Here's how the part is built. I have some questions about the finished solid (model axes, mm). A direction names the side the tool comes from. Round coordinates to 2 decimals unless told otherwise and drop trailing zeros. Write each loop counter-clockwise with the first axis right and the second up, starting at its lowest first coordinate (ties: lowest second). Pieces come first, ordered by that corner, then holes. Notation, with made-up numbers: (2, 35.5) - (29, 35.5) arc R27 cw to (29, 62.5) - close; hole circle Ø5 at (-18, -12). An arc over 180 degrees is marked (long way). One line per item, written item: value. Start each with the question number.
Item 1: For P1, Ø4.5, axis at x = -12.55, y = 36.5, coming from the +Z side; P2, Ø4, axis at x = 18.95, z = 389.69, coming from the +Y side; P3, Ø2.5, axis at y = 75, z = 389.69, coming from the +X side; P4, Ø1, axis at y = 26, z = 388.5, coming from the +X side, each with a flat end and sliding along its axis, tell me the tip position at first contact or that it passes through.
Item 2: Thinking about a two-plate mould opening in Z: for faces 1 (the face through (-1, 49, 384.692)), 2 (the face through (-15.48, 72.6, 389.62)), 3 (the face through (19.144, 15.043, 390)), which applies, released by +Z, released by -Z, zero draft, split by the parting line, or undercut?
Item 3: For faces 4 (the face through (19.892, 25.631, 391.695)), 5 (the face through (18.493, 92.902, 387.642)), 6 (the face through (-17.009, 74.676, 389.86)), 7 (the face through (-15.48, 91.4, 389.62)), 8 (the face through (-26.052, 49, 390)), which set-ups out of +Z, -Z, +X, -X, +Y, -Y let a thin tool reach every point of the face, with its end or its side?
Item 4: Imagine slicing it at C-C, the plane x = 6. Please give me the cut outline in (y, z), then the cut area to 3 significant figures.
Item 5: Imagine slicing it at B-B, the plane z = 393.75. Please give me the cut outline in (x, y).
Item 6: Imagine slicing it at D-D, the plane y = 18.5. Please give me the cut outline in (x, z).
Item 7: If I drill on line 1 (Y direction, x = -1.5, z = 388.75); line 2 (X direction, y = 38, z = 387.25); line 3 (X direction, y = 88, z = 388), over which ranges is the centre line in solid material (lowest first)?
Item 8: Imagine slicing it at A-A, the plane y = 36.5. Please give me the cut outline in (x, z), then the cut area to 3 significant figures.
```python
from build123d import *

# Parameters (mm, degrees)
SKETCH1_W                 = 50
SKETCH1_H                 = 10
BOSS_EXTRUDE1_DEPTH       = 100
M5X0_8_TAPPED_HOLE1_D     = 4.2
M5X0_8_TAPPED_HOLE1_DEPTH = 14
M5X0_8_TAPPED_HOLE1_TIP   = 1.2618073
M5X0_8_TAPPED_HOLE2_D     = 4.2
M5X0_8_TAPPED_HOLE2_DEPTH = 14
M5X0_8_TAPPED_HOLE2_TIP   = 1.2618073
M5X0_8_TAPPED_HOLE3_D     = 4.2
M5X0_8_TAPPED_HOLE3_DEPTH = 8
M5X0_8_TAPPED_HOLE3_TIP   = 1.2618073
M5X0_8_TAPPED_HOLE4_D     = 4.2
M5X0_8_TAPPED_HOLE4_DEPTH = 8
M5X0_8_TAPPED_HOLE4_TIP   = 1.2618073
CUT_EXTRUDE2_REACH        = 12
SKETCH11_R                = 10.5
SKETCH11_R_2              = 1.75
SKETCH11_W                = 30
SKETCH11_H                = 20
FILLET2_R                 = 2


with BuildPart() as part:
    # Sketch1 → Boss-Extrude1 (new body)
    with BuildSketch(Plane(origin=(0, 0, 0), x_dir=(1, 0, 0), z_dir=(0, 1, 0))):
        with Locations((-1.051745534, -389.692172039)):
            Rectangle(SKETCH1_W, SKETCH1_H)
    extrude(amount=BOSS_EXTRUDE1_DEPTH)

    # M5x0.8 Tapped Hole1
    with Locations(Plane.XZ):
        with Locations((18.948254466, 389.692172039), (-21.051745534, 389.692172039)):
            Hole(M5X0_8_TAPPED_HOLE1_D / 2, depth=M5X0_8_TAPPED_HOLE1_DEPTH)
            with Locations((0, 0, -(M5X0_8_TAPPED_HOLE1_DEPTH + M5X0_8_TAPPED_HOLE1_TIP / 2))):  # 118° drill point
                Cone(0, M5X0_8_TAPPED_HOLE1_D / 2, M5X0_8_TAPPED_HOLE1_TIP, mode=Mode.SUBTRACT)

    # M5x0.8 Tapped Hole2
    with Locations(Plane(origin=(0, 100, 0), x_dir=(-1, 0, 0), z_dir=(0, 1, 0))):
        with Locations((21.051745534, 389.692172039), (-18.948254466, 389.692172039)):
            Hole(M5X0_8_TAPPED_HOLE2_D / 2, depth=M5X0_8_TAPPED_HOLE2_DEPTH)
            with Locations((0, 0, -(M5X0_8_TAPPED_HOLE2_DEPTH + M5X0_8_TAPPED_HOLE2_TIP / 2))):  # 118° drill point
                Cone(0, M5X0_8_TAPPED_HOLE2_D / 2, M5X0_8_TAPPED_HOLE2_TIP, mode=Mode.SUBTRACT)

    # M5x0.8 Tapped Hole3
    with Locations(Plane.ZY.offset(26.051745534)):
        with Locations((389.692172039, 75), (389.692172039, 25)):
            Hole(M5X0_8_TAPPED_HOLE3_D / 2, depth=M5X0_8_TAPPED_HOLE3_DEPTH)
            with Locations((0, 0, -(M5X0_8_TAPPED_HOLE3_DEPTH + M5X0_8_TAPPED_HOLE3_TIP / 2))):  # 118° drill point
                Cone(0, M5X0_8_TAPPED_HOLE3_D / 2, M5X0_8_TAPPED_HOLE3_TIP, mode=Mode.SUBTRACT)

    # M5x0.8 Tapped Hole4
    with Locations(Plane(origin=(23.948254466, 0, 0), x_dir=(0, 0, -1), z_dir=(1, 0, 0))):
        with Locations((-389.692172039, 75), (-389.692172039, 25)):
            Hole(M5X0_8_TAPPED_HOLE4_D / 2, depth=M5X0_8_TAPPED_HOLE4_DEPTH)
            with Locations((0, 0, -(M5X0_8_TAPPED_HOLE4_DEPTH + M5X0_8_TAPPED_HOLE4_TIP / 2))):  # 118° drill point
                Cone(0, M5X0_8_TAPPED_HOLE4_D / 2, M5X0_8_TAPPED_HOLE4_TIP, mode=Mode.SUBTRACT)

    # Sketch11 → Cut-Extrude2 (cut, up to next)
    with BuildSketch(Plane.XY.offset(394.692172039), mode=Mode.PRIVATE) as cut_extrude2_sk1:
        with Locations((-1.051745534, 25)):
            Circle(SKETCH11_R)
    cut_extrude2_tool1 = extrude(cut_extrude2_sk1.sketch, amount=-CUT_EXTRUDE2_REACH, mode=Mode.PRIVATE) & part.part
    add(cut_extrude2_tool1.solids().sort_by_distance((-1.051746, 25, 394.692172))[0], mode=Mode.SUBTRACT)
    # Sketch11 → Cut-Extrude2 (cut, up to next)
    with BuildSketch(Plane.XY.offset(394.692172039), mode=Mode.PRIVATE) as cut_extrude2_sk2:
        with Locations((-12.551745534, 36.5)):
            Circle(SKETCH11_R_2)
    cut_extrude2_tool2 = extrude(cut_extrude2_sk2.sketch, amount=-CUT_EXTRUDE2_REACH, mode=Mode.PRIVATE) & part.part
    add(cut_extrude2_tool2.solids().sort_by_distance((-12.551746, 36.5, 394.692172))[0], mode=Mode.SUBTRACT)
    # Sketch11 → Cut-Extrude2 (cut, up to next)
    with BuildSketch(Plane.XY.offset(394.692172039), mode=Mode.PRIVATE) as cut_extrude2_sk3:
        with Locations((10.448254466, 36.5)):
            Circle(SKETCH11_R_2)
    cut_extrude2_tool3 = extrude(cut_extrude2_sk3.sketch, amount=-CUT_EXTRUDE2_REACH, mode=Mode.PRIVATE) & part.part
    add(cut_extrude2_tool3.solids().sort_by_distance((10.448254, 36.5, 394.692172))[0], mode=Mode.SUBTRACT)
    # Sketch11 → Cut-Extrude2 (cut, up to next)
    with BuildSketch(Plane.XY.offset(394.692172039), mode=Mode.PRIVATE) as cut_extrude2_sk4:
        with Locations((10.448254466, 13.5)):
            Circle(SKETCH11_R_2)
    cut_extrude2_tool4 = extrude(cut_extrude2_sk4.sketch, amount=-CUT_EXTRUDE2_REACH, mode=Mode.PRIVATE) & part.part
    add(cut_extrude2_tool4.solids().sort_by_distance((10.448254, 13.5, 394.692172))[0], mode=Mode.SUBTRACT)
    # Sketch11 → Cut-Extrude2 (cut, up to next)
    with BuildSketch(Plane.XY.offset(394.692172039), mode=Mode.PRIVATE) as cut_extrude2_sk5:
        with Locations((-12.551745534, 13.5)):
            Circle(SKETCH11_R_2)
    cut_extrude2_tool5 = extrude(cut_extrude2_sk5.sketch, amount=-CUT_EXTRUDE2_REACH, mode=Mode.PRIVATE) & part.part
    add(cut_extrude2_tool5.solids().sort_by_distance((-12.551746, 13.5, 394.692172))[0], mode=Mode.SUBTRACT)
    # Sketch11 → Cut-Extrude2 (cut, up to next)
    with BuildSketch(Plane.XY.offset(394.692172039), mode=Mode.PRIVATE) as cut_extrude2_sk6:
        with Locations((-1.051745534, 82)):
            Rectangle(SKETCH11_W, SKETCH11_H)
    cut_extrude2_tool6 = extrude(cut_extrude2_sk6.sketch, amount=-CUT_EXTRUDE2_REACH, mode=Mode.PRIVATE) & part.part
    add(cut_extrude2_tool6.solids().sort_by_distance((-1.051746, 82, 394.692172))[0], mode=Mode.SUBTRACT)

    # Fillet2
    fillet2_edges = [part.edges().sort_by_distance(p)[0] for p in [
        (-16.051745534, 72, 389.692172039),
        (-16.051745534, 92, 389.692172039),
        (13.948254466, 92, 389.692172039),
        (13.948254466, 72, 389.692172039),
    ]]
    fillet(fillet2_edges, radius=FILLET2_R)


solid = part.part
```
Values follow:
1. P1: stops at z = 394.69
1. P2: stops at y = 85.94
1. P3: stops at x = 15.44
1. P4: stops at x = 15.92
2. face 1: released by -Z
2. face 2: zero draft
2. face 3: undercut
3. face 4: +X
3. face 5: +Y
3. face 6: -X
3. face 7: +Z, -Z
3. face 8: +Z, -Z, -X, +Y, -Y
4. outline: (0, 384.69) - (17.22, 384.69) - (17.22, 394.69) - (0, 394.69) - close; (32.78, 384.69) - (72, 384.69) - (72, 394.69) - (32.78, 394.69) - close; (92, 384.69) - (100, 384.69) - (100, 394.69) - (92, 394.69) - close
4. area: 644 mm^2
5. outline: (-26.05, 0) - (23.95, 0) - (23.95, 100) - (-26.05, 100) - close; hole (-16.05, 74) arc R2 ccw to (-14.05, 72) - (11.95, 72) arc R2 ccw to (13.95, 74) - (13.95, 90) arc R2 ccw to (11.95, 92) - (-14.05, 92) arc R2 ccw to (-16.05, 90) - close; hole circle Ø3.5 at (-12.55, 13.5); hole circle Ø3.5 at (-12.55, 36.5); hole circle Ø21 at (-1.05, 25); hole circle Ø3.5 at (10.45, 13.5); hole circle Ø3.5 at (10.45, 36.5)
6. outline: (-26.05, 384.69) - (-9.3, 384.69) - (-9.3, 394.69) - (-26.05, 394.69) - close; (7.19, 384.69) - (23.95, 384.69) - (23.95, 394.69) - (7.19, 394.69) - close
7. line 1: y = 0 to 14.51, 35.49 to 72, 92 to 100
7. line 2: x = -26.05 to -13.45, -11.65 to 9.55, 11.35 to 23.95
7. line 3: x = -26.05 to -22.3, -19.81 to -16.05, 13.95 to 17.7, 20.19 to 23.95
8. outline: (-26.05, 384.69) - (-14.3, 384.69) - (-14.3, 394.69) - (-26.05, 394.69) - close; (-10.8, 384.69) - (8.7, 384.69) - (8.7, 394.69) - (-10.8, 394.69) - close; (12.2, 384.69) - (23.95, 384.69) - (23.95, 394.69) - (12.2, 394.69) - close
8. area: 430 mm^2
